Read the model definition and answer for the solid it produces. Units are mm, in the model's axes. Face numbers are marked on the shaded views. A direction names the side the tool comes from. Round coordinates to 2 decimals unless told otherwise and drop trailing zeros. Order: outer loops, then holes, each group sorted by start corner. A loop starts at its lowest first (then second) coordinate and runs counter-clockwise, first axis right, second up. Notation, with made-up numbers: (44.25, 11) - (80.25, 11) arc R19 cw to (80.25, 43) - close; hole circle Ø4 at (-38, 22.25). An arc over 180 degrees is marked (long way). One line per question, with ' | ' between items. Start each with the question number.
1) Flat-ended cylindrical pins translate along their axes: pin 1 (6 mm diameter, centred on y = 4.5, z = 8.5, fed in from -X); pin 2 (12 mm diameter, centred on x = -32, z = 43.5, fed in from +Y); pin 3 (16.5 mm diameter, centred on x = -10.5, z = 40.5, fed in from +Y). Find the tip coordinate at first contact, or state that the pin passes through.
2) Straight lines are drawn through the part: line 1 (Y direction, x = -50, z = 8.5); line 2 (Z direction, x = -6, y = 6.5); line 3 (Z direction, x = -30, y = -4.5). For each, find the intervals that lie inside material, in ascending order. Write a range as from..to.
3) The part is cut by section B-B, the plane y = 0. Give the vertices of the cut face in (x, z).
4) For the marked faces 1, 2, 3, 4 and 5, determine the directions among +Z, -Z, +X, -X, +Y, -Y from which every point of the face is accessible in a straight line to the end or side of a thin tool.
5) The part is cut by section D-D, the plane x = -51.5. Give the vertices of the cut face in (y, z).
6) The part is cut by section C-C, the plane z = 7. Give the vertices of the cut face in (x, y), plus the area to 3 significant figures.
7) The part is cut by section A-A, the plane z = 44. Give the vertices of the cut face in (x, y).
8) The mould has two halves that part along Y. Classify the marked faces 6, 7, 8 and 9: pulls with the +Y half, pulls with the -Y half, needs draft (parallel to the pull), parting line crosses it, or undercut.
from build123d import *

# Parameters (mm, degrees)
F0_R     = 5
F1_DEPTH = 15
F3_DEPTH = 75
F5_DEPTH = 80
F7_DEPTH = 50
F9_DEPTH = 15


with BuildPart() as f1:
    # F0 (on Top) → F1 (new body)
    with BuildSketch(Plane.XY):
        with BuildLine():
            Line((0, 15), (-50, 15))
            ThreePointArc((-50, 15), (-65, 0), (-50, -15))
            Line((-50, -15), (0, -15))
            Line((0, -15), (0, 0))
            Line((0, 0), (0, 15))
        make_face()
        with Locations((-50, 0)):
            Circle(F0_R, mode=Mode.SUBTRACT)
    extrude(amount=F1_DEPTH)

    # F2 (on face) → F3 (join)
    with BuildSketch(Plane(origin=(0, 0, 0), x_dir=(1, 0, 0), z_dir=(0, 0, -1))):
        Polygon((0, -20), (0, -15), (-20, -15), align=None)
        Polygon((0, -15), (0, 0), (0, 15), (-20, 15), (-40, 10), (-40, 0), (-40, -10), (-20, -15), align=None)
        Polygon((-20, 15), (0, 15), (0, 20), align=None)
    extrude(amount=-F3_DEPTH)

    # F4 (on face) → F5 (cut)
    with BuildSketch(Plane.YZ):
        Polygon((34.8571650684, 75), (20, 75), (20, 57.7444738917), (25.7445386642, 51.1361380983), align=None)
        Polygon((20, 75), (5, 75), (20, 57.7444738917), align=None)
        Polygon((-20, 57.7444738917), (-5, 75), (-20, 75), align=None)
        Polygon((-25.7445386642, 51.1361380983), (-20, 57.7444738917), (-20, 75), (-34.8571650684, 75), align=None)
    extrude(amount=-F5_DEPTH, mode=Mode.SUBTRACT)

    # F6 (on face) → F7 (cut)
    with BuildSketch(Plane(origin=(-40, 0, 0), x_dir=(0, -1, 0), z_dir=(-1, 0, 0))):
        with BuildLine():
            Line((5, 42.1240789819), (5, 49.6240789819))
            ThreePointArc((5, 49.6240789819), (0, 54.6240789819), (-5, 49.6240789819))
            Line((-5, 49.6240789819), (-5, 42.1240789819))
            Line((-5, 42.1240789819), (-5, 34.6240789819))
            ThreePointArc((-5, 34.6240789819), (0, 29.6240789819), (5, 34.6240789819))
            Line((5, 34.6240789819), (5, 42.1240789819))
        make_face()
    extrude(amount=-F7_DEPTH, mode=Mode.SUBTRACT)

    # F8 (on face) → F9 (cut)
    with BuildSketch(Plane.YZ):
        with BuildLine():
            Line((15, 34.6240789819), (15, 49.6240789819))
            ThreePointArc((15, 49.6240789819), (0, 64.6240789819), (-15, 49.6240789819))
            Line((-15, 49.6240789819), (-15, 34.6240789819))
            ThreePointArc((-15, 34.6240789819), (0, 19.6240789819), (15, 34.6240789819))
        make_face()
        with BuildLine():
            ThreePointArc((5, 34.6240789819), (0, 29.6240789819), (-5, 34.6240789819))
            Line((-5, 34.6240789819), (-5, 49.6240789819))
            ThreePointArc((-5, 49.6240789819), (0, 54.6240789819), (5, 49.6240789819))
            Line((5, 49.6240789819), (5, 34.6240789819))
        make_face(mode=Mode.SUBTRACT)
    extrude(amount=-F9_DEPTH, mode=Mode.SUBTRACT)


solid = f1.part
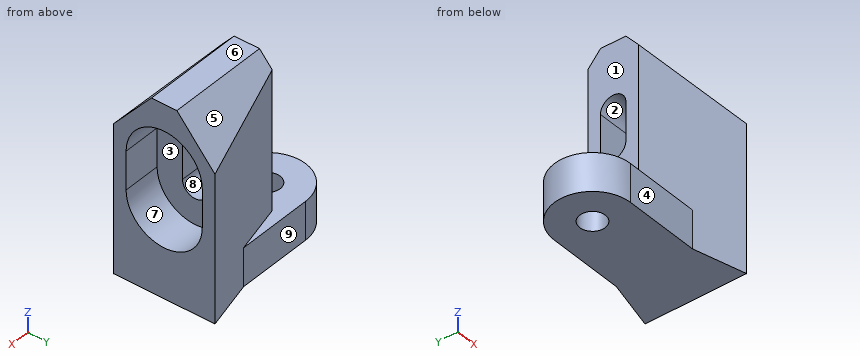
Values:
1) pin 1: stops at x = -64.92 | pin 2: stops at y = 13.5 | pin 3: stops at y = 19.44
2) line 1: y = -15..-5, 5..15 | line 2: z = 0..21.11, 63.14..73.27 | line 3: z = 0..32.44, 51.8..75
3) outline: (-65, 0) - (-55, 0) - (-55, 15) - (-65, 15) - close; (-45, 0) - (0, 0) - (0, 19.62) - (-15, 19.62) - (-15, 29.62) - (-40, 29.62) - (-40, 15) - (-45, 15) - close; (-40, 54.62) - (-15, 54.62) - (-15, 64.62) - (0, 64.62) - (0, 75) - (-40, 75) - close
4) face 1: +Z, -X, +Y, -Y | face 2: +X, -X | face 3: +X | face 4: +Z, -Z, -X, -Y | face 5: +Z, +X, -X, +Y
5) outline: (-14.92, 0) - (-4.77, 0) - (-4.77, 15) - (-14.92, 15) - close; (4.77, 0) - (14.92, 0) - (14.92, 15) - (4.77, 15) - close
6) outline: (-50, -15) - (-20, -15) - (0, -20) - (0, 20) - (-20, 15) - (-50, 15) arc R15 ccw to start; hole circle Ø10 at (-50, 0) | area: 1,870 mm^2
7) outline: (-40, -10) - (0, -20) - (0, -15) - (-15, -15) - (-15, -5) - (-40, -5) - close; (-40, 5) - (-15, 5) - (-15, 15) - (0, 15) - (0, 20) - (-40, 10) - close
8) face 6: needs draft | face 7: undercut | face 8: undercut | face 9: pulls with the +Y half
